```python
from build123d import *

# Parameters (mm, degrees)
F0_W     = 15.8
F0_H     = 7.9
F0_R     = 2.435
F1_DEPTH = 9.6
F2_DEPTH = 11.4
F3_T     = -1.4


# Not quite as in the source:
# - a feature names something its author has since deleted; it is built from what else it names


with BuildPart() as f1:
    # F0 (on Top) → F1 (new body)
    with BuildSketch(Plane.XY):
        with Locations((0, -3.95)):
            Rectangle(F0_W, F0_H)
        with Locations((-3.965, -3.965)):
            Circle(F0_R, mode=Mode.SUBTRACT)
        with Locations((3.965, -3.965)):
            Circle(F0_R, mode=Mode.SUBTRACT)
    extrude(amount=F1_DEPTH)

    # F0 (on Top) → F2 (join)
    with BuildSketch(Plane.XY):
        with Locations((3.965, -3.965)):
            Circle(F0_R)
        with Locations((-3.965, -3.965)):
            Circle(F0_R)
    extrude(amount=F2_DEPTH)

    # F3
    f3_openings = [f1.faces().sort_by_distance(p)[0] for p in [
        (0, -3.95, 0),
    ]]
    offset(amount=F3_T, openings=f3_openings, kind=Kind.INTERSECTION)


solid = f1.part
```
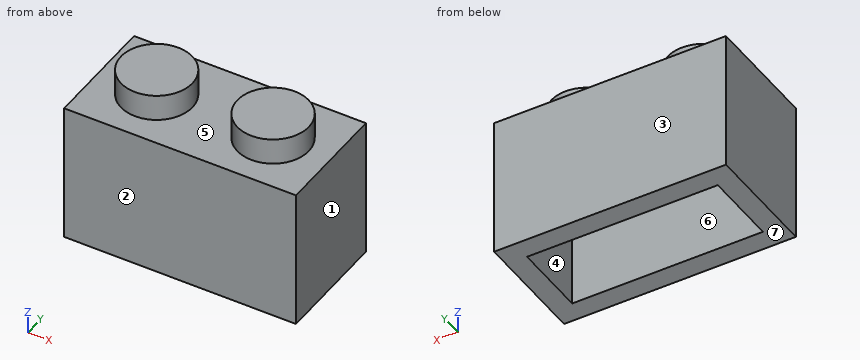
Geometry: final body of the model. Coordinates: model frame, mm. Face numbers are marked on the shaded views. A direction names the side the tool comes from. Round coordinates to 2 decimals unless told otherwise and drop trailing zeros. Loops run counter-clockwise (first coordinate to the right, second up) from the corner with the lowest first, then second, coordinate; pieces in that order, holes last.
Item 1: Contact query for flat-ended pins moving along their axis: P1, Ø1, axis at x = -4, y = -3.5, coming from the -Z side; P2, Ø2.5, axis at x = 4, y = -4, coming from the -Z side. Output: stop coordinate, or through.
Checked values:
P1: stops at z = 10
P2: stops at z = 8.2
Item 2: Section C-C, the plane y = -6. Output: boundary loops of the cut face in (x, z).
Checked values:
outline: (-7.9, 0) - (-6.5, 0) - (-6.5, 8.2) - (6.5, 8.2) - (6.5, 0) - (7.9, 0) - (7.9, 9.6) - (5.3, 9.6) - (5.3, 11.4) - (2.63, 11.4) - (2.63, 9.6) - (-2.63, 9.6) - (-2.63, 11.4) - (-5.3, 11.4) - (-5.3, 9.6) - (-7.9, 9.6) - close
Item 3: Section B-B, the plane x = 1.25. Output: boundary loops of the cut face in (y, z).
Checked values:
outline: (-7.9, 0) - (-6.5, 0) - (-6.5, 8.2) - (-1.4, 8.2) - (-1.4, 0) - (0, 0) - (0, 9.6) - (-7.9, 9.6) - close
Item 4: Section D-D, the plane x = -5.75. Output: boundary loops of the cut face in (y, z).
Checked values:
outline: (-7.9, 0) - (-6.5, 0) - (-6.5, 8.2) - (-1.4, 8.2) - (-1.4, 0) - (0, 0) - (0, 9.6) - (-2.31, 9.6) - (-2.31, 11.4) - (-5.62, 11.4) - (-5.62, 9.6) - (-7.9, 9.6) - close
Item 5: Section A-A, the plane z = 5.75. Output: boundary loops of the cut face in (x, y), plus the area to 3 significant figures.
Checked values:
outline: (-7.9, -7.9) - (7.9, -7.9) - (7.9, 0) - (-7.9, 0) - close; hole (-6.5, -6.5) - (6.5, -6.5) - (6.5, -1.4) - (-6.5, -1.4) - close
area: 58.5 mm2
Item 6: Mould query, pull axis Y, two halves, no side actions, for the marked faces 1, 2, 3 and 4. Classes: released by +Y, released by -Y, zero draft, split by the parting line, or undercut.
Checked values:
face 1: zero draft
face 2: released by -Y
face 3: released by +Y
face 4: undercut
Item 7: Line query: L1, parallel to Y at x = 6, z = 5.25; L2, parallel to X at y = -2.5, z = 1.5; L3, parallel to X at y = -3, z = 11. Output: solid intervals per line, ascending.
Checked values:
L1: y = -7.9 to -6.5, -1.4 to 0
L2: x = -7.9 to -6.5, 6.5 to 7.9
L3: x = -6.2 to -1.73, 1.73 to 6.2
Item 8: Reachability of the marked faces 5, 6 and 7 from +Z, -Z, +X, -X, +Y, -Y: full face, straight path, thin tool, end or side. Return the list, or none.
Checked values:
face 5: +Z
face 6: -Z
face 7: -Z, +X, -X, +Y, -Y
